Read the model definition and answer for the solid it produces. Units are mm, in the model's axes. Give positions to 0.01 mm unless a question says otherwise; leave off trailing zeros. Order: outer loops, then holes, each group sorted by start corner. A loop starts at its lowest first (then second) coordinate and runs counter-clockwise, first axis right, second up.
Autodesk Inventor part; units mm, degrees
ref_plane "YZ Plane" through (0, 0, 0) normal (1, 0, 0) x (0, 1, 0)
ref_plane "XZ Plane" through (0, 0, 0) normal (0, 1, 0) x (-1, 0, 0)
ref_plane "XY Plane" through (0, 0, 0) normal (0, 0, 1) x (1, 0, 0)
sketch "Sketch1" plane through (0, 0, 0) normal (0, 1, 0) x (-1, 0, 0)
  line L0 (0, 0) -> (-82.55, 0)
  line L1 (-82.55, 0) -> (-82.55, 38.1)
  line L2 (-82.55, 38.1) -> (0, 38.1)
  line L3 (0, 38.1) -> (0, 0)
  dimension "d0" = 82.55
  dimension "d1" = 38.1
extrude "Extrusion1" add sketch "Sketch1" along normal blind 3.175
sketch "Sketch2" plane through (0, 3.175, 0) normal (0, 1, 0) x (1, 0, 0)
  line L0 (82.55, 0) -> (0, 0)
  line L1 (0, 0) -> (0, -38.1)
  line L2 (0, -38.1) -> (82.55, -38.1)
  line L3 (82.55, -38.1) -> (82.55, 0)
  line L4 (0, -36.5125) -> (82.55, -36.5125)
  line L5 (82.55, -36.5125) -> (82.55, -33.3121)
  line L6 (82.55, -33.3121) -> (0, -33.3121)
  line L7 (0, -33.3121) -> (0, -36.5125)
  line L8 (1.5875, -3.175) -> (87.3125, -3.175)
  line L9 (87.3125, -3.175) -> (87.3125, -6.604)
  line L10 (87.3125, -6.604) -> (1.5875, -6.604)
  line L11 (1.5875, -6.604) -> (1.5875, -3.175)
  dimension "d4" = 3.2004
  dimension "d5" = 1.5875
  dimension "d8" = 85.725
  dimension "d9" = 1.5875
  dimension "d10" = 3.429
  dimension "d11" = 3.175
extrude "Extrusion2" cut sketch "Sketch2" against normal blind 1.5875 contours L6 L3 L4 L1
sketch "Sketch3" plane through (0, 3.175, 0) normal (0, 1, 0) x (1, 0, 0)
  line L0 (82.55, 0) -> (0, 0)
  line L1 (0, 0) -> (0, -33.3121)
  line L2 (1.5875, -3.175) -> (80.9625, -3.175)
  line L3 (80.9625, -3.175) -> (80.9625, -6.604)
  line L4 (80.9625, -6.604) -> (1.5875, -6.604)
  line L5 (1.5875, -6.604) -> (1.5875, -3.175)
  line L6 (82.55, -33.3121) -> (82.55, 0)
  dimension "d15" = 3.429
  dimension "d16" = 3.175
  dimension "d17" = 1.5875
  dimension "d20" = 1.5875
extrude "Extrusion3" cut sketch "Sketch3" against normal blind 12.7
sketch "Sketch4" plane through (0, 3.175, 0) normal (0, 1, 0) x (1, 0, 0)
  line L0 (0, -38.1) -> (1.5875, -38.1)
  line L1 (1.5875, -38.1) -> (1.5875, -31.75)
  line L2 (1.5875, -31.75) -> (0, -31.75)
  line L3 (0, -31.75) -> (0, -38.1)
  line L4 (82.55, -38.1) -> (80.9625, -38.1)
  line L5 (80.9625, -38.1) -> (80.9625, -31.75)
  line L6 (80.9625, -31.75) -> (82.55, -31.75)
  line L7 (82.55, -31.75) -> (82.55, -38.1)
  point P0 (0, 0)
  dimension "d21" = 1.5875
  dimension "d22" = 6.35
  dimension "d23" = 6.35
  dimension "d24" = 1.5875
extrude "Extrusion4" cut sketch "Sketch4" against normal blind 12.7
fillet "Fillet1" radius 1.5875 2 edges at (80.9625, 1.5875, 31.75) (1.5875, 1.5875, 31.75)
sketch "Sketch5" plane through (0, 3.175, 0) normal (0, 1, 0) x (1, 0, 0)
  line L0 (82.55, -31.75) -> (82.55, 0)
  line L1 (3.2004, 0) -> (79.3496, 0)
  line L2 (79.3496, 0) -> (79.3496, -3.175)
  line L3 (79.3496, -3.175) -> (3.2004, -3.175)
  line L4 (3.2004, -3.175) -> (3.2004, 0)
  line L5 (0, 0) -> (0, -31.75)
  dimension "d31" = 3.175
  dimension "d32" = 3.2004
  dimension "d33" = 3.2004
extrude "Extrusion5" add sketch "Sketch5" along normal blind 19.05
properties part number "Electronics Container Part 5"
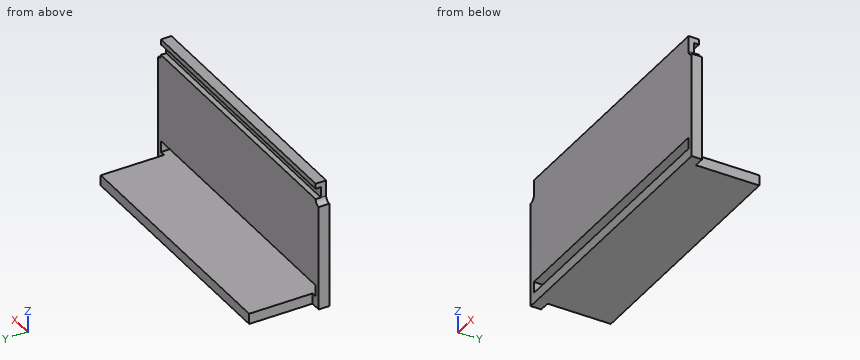
1) The part is cut by section C-C on z = 35.5. Determine the outline of the cut face in (x, y).
Final values:
outline: (1.59, 0) - (80.96, 0) - (80.96, 1.59) - (1.59, 1.59) - close
2) Given pin 1 (2.5 mm diameter, centred on y = 15.5, z = 1, fed in from +X); pin 2 (1 mm diameter, centred on y = 1.5, z = 35.5, fed in from -X); pin 3 (16.5 mm diameter, centred on x = 41, z = 14, fed in from +Y) (3 decimals), each flat-ended and moving along its own axis, determine where each tip first touches the part or whether it passes through.
Final values:
pin 1: stops at x = 79.35
pin 2: stops at x = 1.59
pin 3: stops at y = 3.175
3) The part is cut by section B-B on y = 16. Determine the outline of the cut face in (x, z) (3 decimals).
Final values:
outline: (3.2, 0) - (79.35, 0) - (79.35, 3.175) - (3.2, 3.175) - close
4) The part is cut by section A-A on x = 12. Determine the outline of the cut face in (y, z) (1 decimal).
Final values:
outline: (0, 0) - (22.2, 0) - (22.2, 3.2) - (0, 3.2) - close; (0, 6.6) - (3.2, 6.6) - (3.2, 33.3) - (1.6, 33.3) - (1.6, 36.5) - (3.2, 36.5) - (3.2, 38.1) - (0, 38.1) - close
5) Consider L1, parallel to Z at x = 9.5, y = 2.75 (1 decimal); L2, parallel to Y at x = 55.5, z = 24.5 (3 decimals). Determine where each line is inside the solid, lowest interval first.
Final values:
L1: z = 0 to 3.2, 6.6 to 33.3, 36.5 to 38.1
L2: y = 0 to 3.175
